```python
from build123d import *

# Parameters (mm, degrees)
F0_W            = 18
F0_H            = 10
F1_DEPTH        = 15
F2_W            = 8
F2_H            = 10
F3_DEPTH        = 10
F5_D            = 3.15
F5_CBORE_D      = 6.5
F5_CBORE_DEPTH  = 3
F7_DEPTH        = 2.4
F8_W            = 8
F8_H            = 15
F9_DEPTH        = 17
F10_W           = 8
F10_H           = 8
F11_DEPTH       = 12
F13_D           = 3.15
F13_CSINK_D     = 6.72
F13_CSINK_ANGLE = 90
F15_DEPTH       = 25
F16_R           = 2


with BuildPart() as f1:
    # F0 (on Front) → F1 (new body)
    with BuildSketch(Plane.XZ):
        with Locations((0, 5)):
            Rectangle(F0_W, F0_H)
    extrude(amount=F1_DEPTH)

    # F2 (on face) → F3 (cut)
    with BuildSketch(Plane.XZ.offset(15)):
        with Locations((0, 5)):
            Rectangle(F2_W, F2_H)
    extrude(amount=-F3_DEPTH, mode=Mode.SUBTRACT)

    # F5 (through all)
    with Locations(Plane.YZ.offset(9)):
        with Locations((-10.5, 5)):
            CounterBoreHole(F5_D / 2, F5_CBORE_D / 2, F5_CBORE_DEPTH)

    # F6 (on face) → F7 (cut)
    with BuildSketch(Plane(origin=(-9, 0, 0), x_dir=(0, -1, 0), z_dir=(-1, 0, 0))):
        Polygon((12.1165807537, 2.2), (13.7331615075, 5), (12.1165807537, 7.8), (8.8834192463, 7.8), (7.2668384925, 5), (8.8834192463, 2.2), align=None)
    extrude(amount=-F7_DEPTH, mode=Mode.SUBTRACT)

    # F8 (on face) → F9 (join)
    with BuildSketch(Plane.XZ.offset(5)):
        with Locations((0, 2.5)):
            Rectangle(F8_W, F8_H)
    extrude(amount=-F9_DEPTH)

    # F10 (on face) → F11 (cut, through all)
    with BuildSketch(Plane(origin=(0, 12, 0), x_dir=(-1, 0, 0), z_dir=(0, 1, 0))):
        with Locations((0, -1)):
            Rectangle(F10_W, F10_H)
    extrude(amount=-F11_DEPTH, mode=Mode.SUBTRACT)

    # F13 (through all)
    with Locations(Plane.XZ.offset(5)):
        with Locations((0, -1)):
            CounterSinkHole(F13_D / 2, F13_CSINK_D / 2, counter_sink_angle=F13_CSINK_ANGLE)

    # F14 (on face) → F15 (cut)
    with BuildSketch(Plane(origin=(-4, 0, 0), x_dir=(0, -1, 0), z_dir=(-1, 0, 0))):
        Polygon((-12, 7.8840762315), (0, 10), (-12, 10), align=None)
    extrude(amount=-F15_DEPTH, mode=Mode.SUBTRACT)

    # F16 (call 1 of 3: OpenCascade refuses the feature's edges together)
    f16_edges = [f1.edges().sort_by_distance(p)[0] for p in [
        (-4, -2.5, 0),
    ]]
    fillet(f16_edges, radius=F16_R)

    # F16#2 (call 2 of 3)
    f16_2_edges = [f1.edges().sort_by_distance(p)[0] for p in [
        (0, 0, 3),
        (-4, 0, 6.5),
        (4, 0, 6.5),
        (-4, 6, 3),
        (4, 6, 3),
    ]]
    fillet(f16_2_edges, radius=F16_R)

    # F16#3 (call 3 of 3)
    f16_3_edges = [f1.edges().sort_by_distance(p)[0] for p in [
        (4, -2.5, 0),
    ]]
    fillet(f16_3_edges, radius=F16_R)


solid = f1.part
```
Check sheet for the modelled part. Datum: model origin and axes. Units: mm. A direction names the side the tool comes from. Give positions to 0.01 mm unless a question says otherwise; leave off trailing zeros. Loops run counter-clockwise (first coordinate to the right, second up) from the corner with the lowest first, then second, coordinate; pieces in that order, holes last. Notation, with made-up numbers: M 26,44 L 59,44 A19 ccw 59,54 Z; hole C 72,80.25 d2. An arc over 180 degrees is marked long. Answer as CSV lines item,"result".
Item 1: Sectioned sample at C-C, the plane z = -1. Enter the section's corners in (x, y) (3 decimals), then the cut area to 3 significant figures.
Reply:
outline,"M -4.268,-5 L -3.36,-5 L -1.575,-3.215 L -1.575,0 L -4.268,0 Z; M 1.575,-3.215 L 3.36,-5 L 4.268,-5 L 4.268,0 L 1.575,0 Z"
area,"23.7 mm^2"
Item 2: Set-up check for faces 4 (the face through (6, -9, 0)), 5 (the face through (-4, -9, 6)), 6 (the face through (3.4, 6.93, 3.57)), 7 (the face through (-7.817, -8.064, 3.62)), 8 (the face through (-3.43, 6.93, 3.6)): record each of +Z, -Z, +X, -X, +Y, -Y from which the full face is reachable in a straight line by a thin tool's end or side.
Reply:
face 4,"-Z, +X, -Y"
face 5,"+Z, -Z, -Y"
face 6,"-Z, +X, +Y"
face 7,"-X"
face 8,"-Z, -X, +Y"
Item 3: Draft check along Z on faces 1 (the face through (7.521, -13.747, 5.143)), 2 (the face through (0, 7, 3)), 3 (the face through (0, -4, 10)). Enter one of: pulls with the +Z half, pulls with the -Z half, needs draft (parallel to the pull), parting line crosses it, or undercut.
Reply:
face 1,"undercut"
face 2,"pulls with the -Z half"
face 3,"pulls with the +Z half"
Item 4: Depth check by flat-ended pin: pin 1 Ø1.5 at (x, y) = (-7.5, -11) entering from -Z; pin 2 Ø3 at (y, z) = (-11, 3.5) entering from +X; pin 3 Ø3 at (x, y) = (-0.5, 7.5) entering from -Z; pin 4 Ø1.9 at (x, z) = (0, -1) entering from +Y. Enter the tip coordinate at first touch or a pass-through.
Reply:
pin 1,"z = 0"
pin 2,"x = 6"
pin 3,"z = 3"
pin 4,"through"
Item 5: Sectioned sample at D-D, the plane y = 6.25. Enter the section's corners in (x, z), then the cut area to 3 significant figures.
Reply:
outline,"M -4,5 A2 ccw -2,3 L 2,3 A2 ccw 4,5 L 4,8.9 L -4,8.9 Z"
area,"45.5 mm^2"
Item 6: Sectioned sample at A-A, the plane x = 0. Enter the section's corners in (y, z) (3 decimals), then the cut area to 3 significant figures.
Reply:
outline,"M -5,-5 L 0,-5 L 0,-2.575 L -3.215,-2.575 L -5,-4.36 Z; M -5,2.36 L -3.215,0.575 L 0,0.575 L 0,1 A2 cw 2,3 L 12,3 L 12,7.884 L 0,10 L -5,10 Z"
area,"128 mm^2"
Item 7: Sectioned sample at B-B, the plane y = -10.5. Enter the section's corners in (x, z) (3 decimals).
Reply:
outline,"M -9,0 L -4,0 L -4,3.425 L -6.6,3.425 L -6.6,2.2 L -9,2.2 Z; M -9,7.8 L -6.6,7.8 L -6.6,6.575 L -4,6.575 L -4,10 L -9,10 Z; M 4,0 L 9,0 L 9,1.75 L 6,1.75 L 6,3.425 L 4,3.425 Z; M 4,6.575 L 6,6.575 L 6,8.25 L 9,8.25 L 9,10 L 4,10 Z"
Item 8: Scan lines: L1, parallel to X at y = -11.25, z = 2.25; L2, parallel to Z at x = 5.15, y = -10.5 (3 decimals); L3, parallel to Y at x = 2.5, z = 3.75. Record each from-to range of solid material in increasing order.
Reply:
L1,"-6.6 to -4, 4 to 6"
L2,"0 to 3.425, 6.575 to 10"
L3,"-5 to 12"
